Source: CAD feature listing. Evaluate the final solid. Frame: model axes, mm. Give positions to 0.01 mm unless a question says otherwise; leave off trailing zeros. Loops run counter-clockwise (first coordinate to the right, second up) from the corner with the lowest first, then second, coordinate; pieces in that order, holes last. Notation, with made-up numbers: M -3,32.5 L 4,32.5 A20 cw 4,60.5 Z; hole C 39,48 d10. An arc over 180 degrees is marked long. Answer in a Markdown table with one row per item.
```python
from build123d import *

# Parameters (mm, degrees)
F0_W     = 8
F0_H     = 4
F1_DEPTH = 28
F2_SIZE2 = 1
F2_SIZE  = 5


with BuildPart() as f1:
    # F0 (on Top) → F1 (new body)
    with BuildSketch(Plane.XY):
        with Locations((-11.080092, -2)):
            Rectangle(F0_W, F0_H)
    extrude(amount=F1_DEPTH)

    # F2
    f2_edges = [f1.edges().sort_by_distance(p)[0] for p in [
        (-11.080092, 0, 28),
        (-11.080092, -4, 28),
        (-7.080092, -2, 28),
        (-15.080092, -2, 28),
    ]]
    chamfer(f2_edges, length=F2_SIZE, length2=F2_SIZE2)


solid = f1.part
```
1) Section C-C, the plane z = 24.5. Return loops of the section in (x, y), then the cut area to 3 significant figures.
Reply:
| item | result |
|---|---|
| outline | M -14.78,-3.7 L -7.38,-3.7 L -7.38,-0.3 L -14.78,-0.3 Z |
| area | 25.2 mm² |
2) Material intervals for L1, parallel to X at y = -2.25, z = 25.5; L2, parallel to Y at x = -9.25, z = 27.25, sorted ascending.
Reply:
| item | result |
|---|---|
| L1 | x = -14.58 to -7.58 |
| L2 | y = -3.15 to -0.85 |
3) Section A-A, the plane x = -11.25. Return loops of the section in (y, z), then the cut area to 3 significant figures.
Reply:
| item | result |
|---|---|
| outline | M -4,0 L 0,0 L 0,23 L -1,28 L -3,28 L -4,23 Z |
| area | 107 mm² |
4) Section B-B, the plane y = -0.4. Return loops of the section in (x, z).
Reply:
| item | result |
|---|---|
| outline | M -15.08,0 L -7.08,0 L -7.08,23 L -7.48,25 L -14.68,25 L -15.08,23 Z |
